from build123d import *

# Parameters (mm, degrees)
SKETCH1_R           = 12
BOSS_EXTRUDE1_DEPTH = 11.59
EXTRUDE_THIN2_START = -4.1
SKETCH8_R           = 10.5
SKETCH8_R_2         = 10
EXTRUDE_THIN2_DEPTH = 22
SKETCH3_R           = 10.5
SKETCH3_R_2         = 10
EXTRUDE_THIN1_DEPTH = 22
SKETCH4_R           = 7.5
CUT_EXTRUDE1_DEPTH  = 10
SKETCH5_R           = 3
CUT_EXTRUDE2_DEPTH  = 24.1800001


with BuildPart() as part:
    # Sketch1 → Boss-Extrude1 (new body, symmetric)
    with BuildSketch(Plane.XY):
        Circle(SKETCH1_R)
    extrude(amount=BOSS_EXTRUDE1_DEPTH, both=True)

    # Sketch8 → Extrude-Thin2 (add)
    with BuildSketch(Plane(origin=(0, 0, 0), x_dir=(-0.342020143, 0.939692621, 0), z_dir=(0.925416578, 0.336824089, -0.173648178)).offset(EXTRUDE_THIN2_START)):
        with Locations((0, -1.5)):
            Circle(SKETCH8_R)
        with Locations((0, -1.5)):
            Circle(SKETCH8_R_2, mode=Mode.SUBTRACT)
    extrude(amount=-EXTRUDE_THIN2_DEPTH)

    # Sketch3 → Extrude-Thin1 (add)
    with BuildSketch(Plane(origin=(0, 0, 0), x_dir=(0, 0, -1), z_dir=(0.939692621, -0.342020143, 0))):
        Circle(SKETCH3_R)
        Circle(SKETCH3_R_2, mode=Mode.SUBTRACT)
    extrude(amount=EXTRUDE_THIN1_DEPTH)

    # Sketch4 → Cut-Extrude1 (cut)
    with BuildSketch(Plane(origin=(0, 0, -11.59), x_dir=(-1, 0, 0), z_dir=(0, 0, -1))):
        Circle(SKETCH4_R)
    extrude(amount=-CUT_EXTRUDE1_DEPTH, mode=Mode.SUBTRACT)

    # Sketch5 → Cut-Extrude2 (cut, through all)
    with BuildSketch(Plane.XY.offset(11.59)):
        Circle(SKETCH5_R)
    extrude(amount=-CUT_EXTRUDE2_DEPTH, mode=Mode.SUBTRACT)


solid = part.part
Geometry: final body of the model. Coordinates: model frame, mm. A direction names the side the tool comes from. Give positions to 0.01 mm unless a question says otherwise; leave off trailing zeros. Write each loop counter-clockwise with the first axis right and the second up, starting at its lowest first coordinate (ties: lowest second). Pieces come first, ordered by that corner, then holes.
(1) First-contact query: P1, Ø4.5, axis at x = -3, y = 3.5, coming from the -Z side; P2, Ø8, axis at x = -10.5, y = -12.5, coming from the +Z side; P3, Ø7, axis at x = 0, y = 5.5, coming from the +Z side. Flat tips, straight axial feed; report the tip coordinate or a pass-through.
(2) Ray query, line 1 (Z direction, x = 18.5, y = -7); line 2 (Y direction, x = 0, z = -4.75); line 3 (Y direction, x = 0, z = 5). Return the intervals inside material, ascending.
(3) Mould query, pull axis Z, two halves, no side actions, for faces 1 (the cylindrical face through (-3, 0, 5)), 2 (the cylindrical face through (15.11, -5.03, 9.99)), 3 (the flat face through (-3.2, 0.1, -1.59)). Classes: released by +Z, released by -Z, zero draft, split by the parting line, or undercut.
(4) Access query for faces 4 (the cylindrical face through (7.493, 0.33, -6.66)), 5 (the cylindrical face through (-1.56, 11.9, 0.16)), 6 (the flat face through (5, 6, -11.59)), 7 (the flat face through (2.5, -2.5, 11.59)). Directions: +Z, -Z, +X, -X, +Y, -Y. A direction counts if a zero-diameter tool reaches every point of the face in a straight line with its end or side. Return the directions, or none.
(5) Cut plane B-B, the plane x = 10. Give the number of separate pieces and of enclosed holes in the cut face, then the cut area to 3 significant figures.
(6) Cut plane A-A, the plane x = 0. Return loops of the section in (y, z).
Values follow:
1. P1: stops at z = -1.59
1. P2: stops at z = 10.89
1. P3: stops at z = 11.59
2. line 1: z = -10.5 to -10, 10 to 10.5
2. line 2: y = -12 to -7.5, 7.5 to 12
2. line 3: y = -12 to -3, 3 to 12
3. face 1: zero draft
3. face 2: undercut
3. face 3: released by -Z
4. face 4: -Z
4. face 5: none
4. face 6: -Z, +X, -X, +Y, -Y
4. face 7: +Z, +X, +Y, -Y
5. separate pieces: 1
5. enclosed holes: 2
5. area: 325 mm2
6. outline: (-12, -11.59) - (-7.5, -11.59) - (-7.5, -1.59) - (-3, -1.59) - (-3, 11.59) - (-12, 11.59) - close; (3, -1.59) - (7.5, -1.59) - (7.5, -11.59) - (12, -11.59) - (12, 11.59) - (3, 11.59) - close
